Can you work these out from the model? Positions are in its coordinate system, mm. Face numbers are marked on the shaded views. Coordinates: 2 decimals unless noted, no trailing zeros. Loops run counter-clockwise (first coordinate to the right, second up) from the corner with the lowest first, then second, coordinate; pieces in that order, holes last.
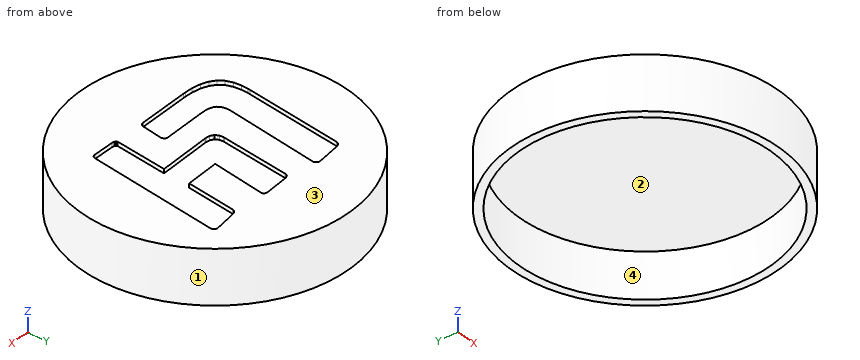
```python
from build123d import *

# Parameters (mm, degrees)
F0_R     = 32.5
F1_DEPTH = 2
F2_R     = 32.5
F2_R_2   = 30.5
F3_DEPTH = 11
F5_START = 1
F5_DEPTH = 2


with BuildPart() as f1:
    # F0 (on Top) → F1 (new body)
    with BuildSketch(Plane.XY):
        Circle(F0_R)
    extrude(amount=F1_DEPTH)

    # F2 (on Top) → F3 (join)
    with BuildSketch(Plane.XY):
        Circle(F2_R)
        Circle(F2_R_2, mode=Mode.SUBTRACT)
    extrude(amount=-F3_DEPTH)

    # F4 (on Top) → F5 (cut)
    with BuildSketch(Plane.XY.offset(F5_START)):
        Polygon((2.4237075291, -15.8480604819), (2.4399934727, -15.7433961512), (3.0970268987, -11.0418947956), (3.1142315365, -10.9209111143), (3.0897608623, -10.5466517793), (2.9266508736, -10.1506277423), (2.6207256875, -9.8973353851), (2.2931694276, -9.820766395), (2.1871855179, -9.8289177185), (-8.2267149419, -10.3341410951), (-8.495391252, -10.347278423), (-9.3028399824, -10.3323204102), (-10.2167737285, -10.2068184235), (-10.9685161801, -9.9476297195), (-11.5570651254, -9.5443730532), (-11.9825708962, -8.9865836618), (-12.2435635816, -8.2651915276), (-12.340068237, -7.3698822195), (-12.305633906, -6.5574224295), (-12.2711995751, -6.290082402), (-9.4904206453, 16.2064848687), (-9.4823194323, 16.3074577188), (-9.5656700563, 16.6188115528), (-9.8257440475, 16.9269081981), (-10.2090901038, 17.1022952827), (-10.5461673769, 17.1344495816), (-10.6535710868, 17.1163262495), (-16.1638908625, 16.3583199734), (-16.2830538588, 16.3401131236), (-16.6314978853, 16.2273642835), (-17.0234379088, 15.9915939313), (-17.3011925884, 15.6618662122), (-17.4190109504, 15.3519321784), (-17.4276216211, 15.2458647511), (-19.9550747867, -8.4637130038), (-20.0121674586, -8.991110319), (-20.0411731417, -10.5892457856), (-19.799205779, -12.4161945835), (-19.2178644077, -13.944542694), (-18.2871686674, -15.1747327606), (-16.9962529107, -16.105887848), (-15.3346857818, -16.7384255445), (-13.2911506379, -17.0728219007), (-11.463274794, -17.1344495816), (-10.8556838224, -17.1086175695), (1.3783169873, -16.6029515493), (1.4797909433, -16.6029515493), (1.7857161295, -16.5608085384), (2.0987403167, -16.4194381965), (2.3167214075, -16.1548208447), align=None)
        Polygon((-3.0113711872, 14.8960092761), (-3.0200570238, 14.7909440607), (-4.687821163, -1.6389839538), (-4.7205600855, -1.93705848), (-4.6257675421, -2.8528296145), (-4.1513872371, -3.6924326438), (-3.2878146396, -4.1628041012), (-2.3643598804, -4.2841552602), (-2.0593533885, -4.2678693166), (10.6803468484, -3.5093619345), (9.4668352583, -15.8444441673), (9.4587340453, -15.9377751516), (9.5180315834, -16.2264121822), (9.7255729669, -16.476079873), (10.0568040038, -16.6120132154), (10.3725842737, -16.6532458838), (10.4782341128, -16.6532458838), (15.4827792953, -16.5521978678), (15.5716420848, -16.5521978678), (15.8388985947, -16.5100632086), (16.1335488968, -16.3686845149), (16.3428441511, -16.1040671631), (16.4352982, -15.7964048096), (16.4433994129, -15.6926508214), (20.0325708227, 16.1054285009), (20.0411731417, 16.1955440553), (19.9804558033, 16.4750776611), (19.7670681837, 16.7878512953), (19.4208039681, 16.9872079482), (19.0796343298, 17.0319734136), (18.9708108197, 17.0152698817), (13.9154869003, 16.2064848687), (13.7822762336, 16.1888626426), (13.3884904699, 16.0890590397), (12.9612976424, 15.8715790548), (12.6567922565, 15.5313281107), (12.5163155535, 15.1688614692), (12.4999460922, 15.0438355331), (11.2363239065, 3.2143942653), (3.0970268987, 2.7086948381), (4.7653756615, 15.4986727059), (4.7811604991, 15.5943004258), (4.7345576452, 15.896049729), (4.5189150488, 16.1752492641), (4.1609583609, 16.3305921105), (3.8165315338, 16.3668387746), (3.703699176, 16.3583199734), (-1.9076853192, 15.8525370285), (-2.0253617012, 15.8444358155), (-2.3728786817, 15.7505619664), (-2.7105405783, 15.5304094164), (-2.9243457862, 15.2060268276), align=None)
    extrude(amount=F5_DEPTH, mode=Mode.SUBTRACT)


solid = f1.part
```
Item 1: Suppose I cut it at D-D, the plane y = -24. Please give me the cut outline in (x, z), plus the area to 3 significant figures.
Results are:
outline: (-21.91, -11) - (-18.82, -11) - (-18.82, 0) - (18.82, 0) - (18.82, -11) - (21.91, -11) - (21.91, 2) - (-21.91, 2) - close
area: 156 mm2
Item 2: Suppose I cut it at C-C, the plane x = 0. Please give me the cut outline in (y, z), plus the area to 3 significant figures.
Results are:
outline: (-32.5, -11) - (-30.5, -11) - (-30.5, 0) - (30.5, 0) - (30.5, -11) - (32.5, -11) - (32.5, 2) - (16.02, 2) - (16.02, 1) - (-4.15, 1) - (-4.15, 2) - (-9.94, 2) - (-9.94, 1) - (-16.66, 1) - (-16.66, 2) - (-32.5, 2) - close
area: 147 mm2
Item 3: I'm going to push flat-ended pins straight in: P1, Ø1.5, axis at x = 23.5, z = -9, coming from the +Y side; P2, Ø1.5, axis at x = -21.5, z = -2.5, coming from the +Y side; P3, Ø6, axis at x = -2.5, z = -5.5, coming from the -Y side. Where does each tip first touch, or does it pass through?
Results are:
P1: stops at y = 23.21
P2: stops at y = 25.01
P3: stops at y = -32.5
Item 4: Suppose I cut it at B-B, the plane y = 8.5. Please give me the cut outline in (x, z), plus the area to 3 significant figures.
Results are:
outline: (-31.37, -11) - (-29.29, -11) - (-29.29, 0) - (29.29, 0) - (29.29, -11) - (31.37, -11) - (31.37, 2) - (19.17, 2) - (19.17, 1) - (11.8, 1) - (11.8, 2) - (3.85, 2) - (3.85, 1) - (-3.66, 1) - (-3.66, 2) - (-10.44, 2) - (-10.44, 1) - (-18.15, 1) - (-18.15, 2) - (-31.37, 2) - close
area: 149 mm2
Item 5: We'd pull the mould along X, two halves only. Please class the marked faces 1, 2, 3 and 4: +X half, -X half, draft (parallel to the pull), parting line (faces both ways), or undercut.
Results are:
face 1: parting line
face 2: undercut
face 3: draft
face 4: undercut
Item 6: Suppose I cut it at A-A, the plane z = -8.25. Please give me the cut outline in (x, y).
Results are:
outline: circle Ø65 at (0, 0); hole circle Ø61 at (0, 0)
Item 7: I need wall thicknesses on line 1 along Y through (x, z) = (0, -8.5); line 2 along Z through (x, y) = (-9.5, 2); line 3 along Y through (x, z) = (14, -0.75). Which ranges of each line are inside material? Lowest first, please.
Results are:
line 1: y = -32.5 to -30.5, 30.5 to 32.5
line 2: z = 0 to 2
line 3: y = -29.33 to -27.1, 27.1 to 29.33
